Geometry check sheet. Reference: the model listing, model coordinates, mm. A direction names the side the tool comes from. Give positions to 0.01 mm unless a question says otherwise; leave off trailing zeros. Write each loop counter-clockwise with the first axis right and the second up, starting at its lowest first coordinate (ties: lowest second). Pieces come first, ordered by that corner, then holes. Notation, with made-up numbers: (53, 13) - (72, 13) arc R18 cw to (72, 42) - close; hole circle Ø8 at (89, 87). An arc over 180 degrees is marked (long way). Use a Markdown table: item, result.
```python
from build123d import *

# Parameters (mm, degrees)
EXTRUDE_1_DEPTH     = 5
SKETCH_8_OUTSIDE_W  = 22.464
SKETCH_8_OUTSIDE_H  = 20.522
SKETCH_8_OUTSIDE_R  = 6.278684177
CUT_EXTRUDE_1_DEPTH = 1
CUT_EXTRUDE_1_DRAFT = -45
SKETCH_9_R          = 3.825
BOLT_LENGTH_DEPTH   = 40
FILLET_1_R          = 1
CHAMFER_1_SIZE      = 1


with BuildPart() as part:
    # Эскиз6 → Бобышка-Вытянуть1 (new body)
    with BuildSketch(Plane(origin=(0, 0, 0), x_dir=(1, 0, 0), z_dir=(0, 1, 0))):
        Polygon((7.25, 0), (3.625, 6.278684177), (-3.625, 6.278684177), (-7.25, 0), (-3.625, -6.278684177), (3.625, -6.278684177), align=None)
    extrude(amount=EXTRUDE_1_DEPTH)


with BuildPart() as cut_extrude_1_tool:
    # Эскиз8 outside → Вырез-Вытянуть1 (with draft: the straight prism first)
    with BuildSketch(Plane(origin=(0, 5, 0), x_dir=(1, 0, 0), z_dir=(0, 1, 0))):
        Rectangle(SKETCH_8_OUTSIDE_W, SKETCH_8_OUTSIDE_H)
        Circle(SKETCH_8_OUTSIDE_R, mode=Mode.SUBTRACT)
    extrude(amount=-CUT_EXTRUDE_1_DEPTH)
    # Вырез-Вытянуть1: the draft: its side faces are tilted about the plane it starts from
    cut_extrude_1_sides = [cut_extrude_1_tool.faces().sort_by_distance(p)[0] for p in [
        (0, 4.5, 10.261),
        (11.232, 4.5, 0),
        (0, 4.5, -10.261),
        (-11.232, 4.5, 0),
        (-6.278684177, 4.5, 0),
    ]]
    draft(cut_extrude_1_sides, Plane(origin=(0, 5, 0), x_dir=(1, 0, 0), z_dir=(0, 1, 0)), CUT_EXTRUDE_1_DRAFT)


with BuildPart() as part_1:
    add(part.part)

    # Вырез-Вытянуть1: cut by cut_extrude_1_tool
    add(cut_extrude_1_tool.part, mode=Mode.SUBTRACT)

    # Эскиз9 → bolt length (add)
    with BuildSketch(Plane.XZ):
        with Locations(Location((0, 0, 0), (0, 0, 90))):  # turned: the seam where the file's is
            Circle(SKETCH_9_R)
    extrude(amount=BOLT_LENGTH_DEPTH)

    # Скругление1
    fillet_1_edges = [part_1.edges().sort_by_distance(p)[0] for p in [
        (0, 0, -3.825),
    ]]
    fillet(fillet_1_edges, radius=FILLET_1_R)

    # Фаска1
    chamfer_1_edges = [part_1.edges().sort_by_distance(p)[0] for p in [
        (0, -40, -3.825),
    ]]
    chamfer(chamfer_1_edges, length=CHAMFER_1_SIZE)


solid = part_1.part
```
1) Material ranges on L1, parallel to X at y = -14.5, z = -1.25; L2, parallel to Y at x = -5.5, z = -0.75; L3, parallel to Z at x = -0.25, y = -2, recorded low to high. Write a range as from..to.
Working result:
| item | result |
|---|---|
| L1 | x = -3.61..3.61 |
| L2 | y = 0..5 |
| L3 | z = -3.82..3.82 |
2) Set-up check for faces 1 (the conical face through (6.51, 4.77, 0.02)), 2 (the cylindrical face through (2.327, -19.734, -3.035)): record each of +Z, -Z, +X, -X, +Y, -Y from which the full face is reachable in a straight line by a thin tool's end or side.
Working result:
| item | result |
|---|---|
| face 1 | +X, +Y |
| face 2 | -Y |
3) Depth check by flat-ended pin: P1, Ø4, axis at x = 1.5, z = -5, coming from the -Y side; P2, Ø3, axis at y = -15.5, z = 1, coming from the -X side (3 decimals); P3, Ø5, axis at x = 0.5, y = -18, coming from the -Z side (3 decimals). Enter the tip coordinate at first touch or a pass-through.
Working result:
| item | result |
|---|---|
| P1 | stops at y = -39.6 |
| P2 | stops at x = -3.825 |
| P3 | stops at z = -3.825 |
4) Section check A-A on y = 1. Record the boundary of the cut face in (x, z) (3 decimals), then the cut area to 3 significant figures.
Working result:
| item | result |
|---|---|
| outline | (-7.25, 0) - (-3.625, -6.279) - (3.625, -6.279) - (7.25, 0) - (3.625, 6.279) - (-3.625, 6.279) - close |
| area | 137 mm² |
5) Section check B-B on y = -10. Record the boundary of the cut face in (x, z) (3 decimals).
Working result:
| item | result |
|---|---|
| outline | circle Ø7.65 at (0, 0) |
